Design review of the part shown in the three views and the two pictorial views. Dimensions are in mm from the part's minimum x, y and z. A direction names the side the tool comes from. Give positions to 0.01 mm unless a question says otherwise; leave off trailing zeros. Loops run counter-clockwise (first coordinate to the right, second up) from the corner with the lowest first, then second, coordinate; pieces in that order, holes last. Notation, with made-up numbers: (-28, 86.25) - (26, 86.25) arc R5 ccw to (26, 95.25) - close; hole circle Ø2 at (-20.75, 15). An arc over 180 degrees is marked (long way). Answer as a JSON object with one key per item and string values.
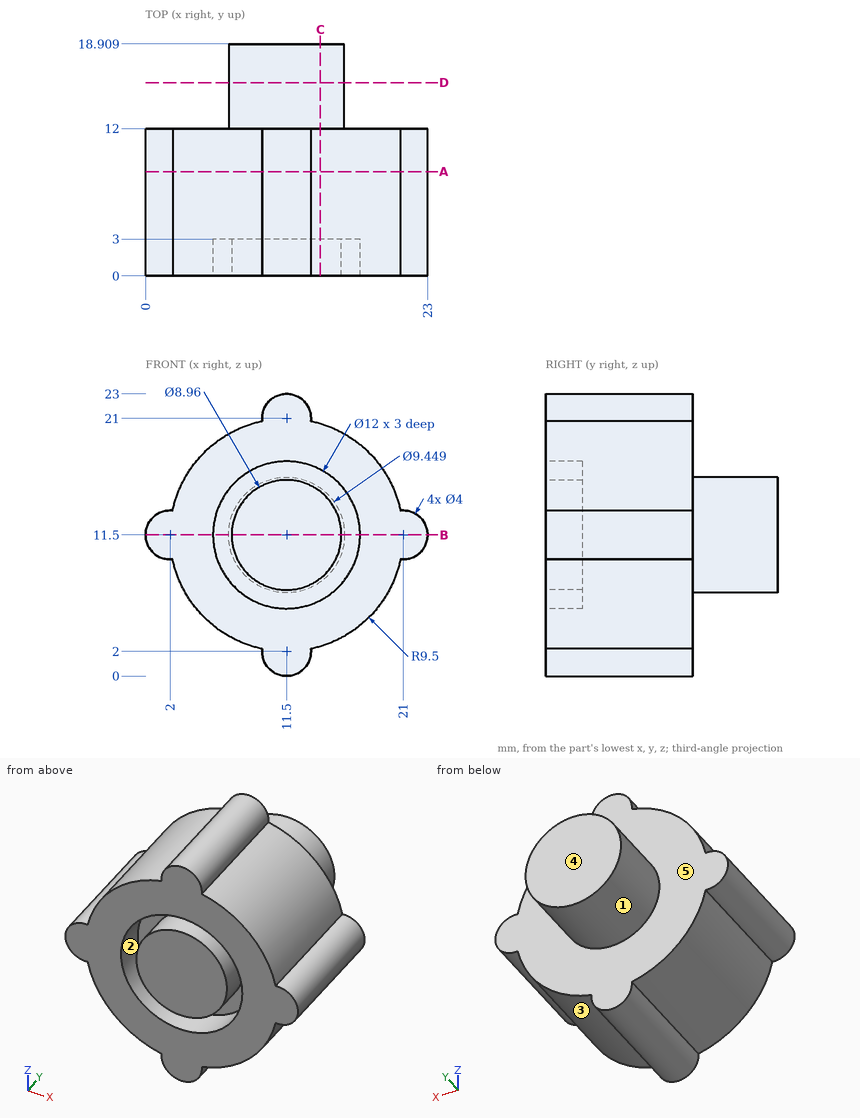
Q1. Consider section B-B, the plane z = 11.5. State the section outline as (x, y) points, plus the area to 3 significant figures.
Results:
{"outline": "(0, 0) - (5.5, 0) - (5.5, 3) - (7.02, 3) - (7.02, 0) - (15.98, 0) - (15.98, 3) - (17.5, 3) - (17.5, 0) - (23, 0) - (23, 12) - (16.22, 12) - (16.22, 18.91) - (6.78, 18.91) - (6.78, 12) - (0, 12) - close", "area": "332 mm^2"}
Q2. Consider section C-C, the plane x = 14.25. State the section outline as (y, z) points.
Results:
{"outline": "(0, 2.41) - (12, 2.41) - (12, 7.66) - (18.91, 7.66) - (18.91, 15.34) - (12, 15.34) - (12, 20.59) - (0, 20.59) - (0, 16.83) - (3, 16.83) - (3, 15.04) - (0, 15.04) - (0, 7.96) - (3, 7.96) - (3, 6.17) - (0, 6.17) - close"}
Q3. For the marked faces 4 and 5, list the 3-axis set-ups (+Z, -Z, +X, -X, +Y, -Y) from which the entire face can be reached by the end or side of a thin tool; tool diameter is ignored.
Results:
{"face 4": "+Z, -Z, +X, -X, +Y", "face 5": "+Y"}
Q4. Clearance check with flat-ended pins moving along their axes: pin 1 Ø8 at (y, z) = (15, 6.5) entering from -X; pin 2 Ø4 at (x, z) = (3.5, 20.5) entering from +Y; pin 3 Ø1 at (y, z) = (5, 5.5) entering from -X. State where each tip first meets the part, or that it passes through.
Results:
{"pin 1": "stops at x = 2.3", "pin 2": "passes through", "pin 3": "stops at x = 3.75"}
Q5. The part is to be moulded in two halves that separate along X. For the marked faces 1, 2 and 3, say which applies: +X half, -X half, draft (parallel to the pull), parting line (faces both ways), or undercut.
Results:
{"face 1": "parting line", "face 2": "undercut", "face 3": "+X half"}
Q6. Consider section D-D, the plane y = 15.75. State the section outline as (x, z) points, plus the area to 3 significant figures.
Results:
{"outline": "circle Ø9.45 at (11.5, 11.5)", "area": "70.1 mm^2"}
Q7. Consider section A-A, the plane y = 8.5. State the section outline as (x, z) points.
Results:
{"outline": "(2.21, 9.51) arc R9.5 ccw to (9.51, 2.21) arc R2 ccw (long way) to (13.49, 2.21) arc R9.5 ccw to (20.79, 9.51) arc R2 ccw (long way) to (20.79, 13.49) arc R9.5 ccw to (13.49, 20.79) arc R2 ccw (long way) to (9.51, 20.79) arc R9.5 ccw to (2.21, 13.49) arc R2 ccw (long way) to start"}
Q8. To check wall thickness, follow probe 1 along Z at (x, y) = (11.5, 1.5); probe 2 along X at (y, z) = (2.75, 16.25) (1 decimal); probe 3 along Y at (x, z) = (15.25, 7.5). State the ranges of each line that lie inside material, in increasing order. Write a range as [from, to].
Results:
{"probe 1": "z = [0, 5.5], [7.02, 15.98], [17.5, 23]", "probe 2": "x = [3.3, 7.8], [15.2, 19.7]", "probe 3": "y = [3, 12]"}
